Build history of the part. All positions in model axes, mm. A direction names the side the tool comes from. Coordinates: 2 decimals unless noted, no trailing zeros. Write each loop counter-clockwise with the first axis right and the second up, starting at its lowest first coordinate (ties: lowest second). Pieces come first, ordered by that corner, then holes.
Autodesk Inventor part; units mm, degrees
ref_plane "YZ Plane" through (0, 0, 0) normal (1, 0, 0) x (0, 1, 0)
ref_plane "XZ Plane" through (0, 0, 0) normal (0, 1, 0) x (-1, 0, 0)
ref_plane "XY Plane" through (0, 0, 0) normal (0, 0, 1) x (1, 0, 0)
sketch "Sketch1" plane through (0, 0, 0) normal (0, 0, 1) x (1, 0, 0)
  line L0 (0, 0) -> (63.5, 0)
  line L1 (63.5, 0) -> (63.5, 127)
  line L2 (63.5, 127) -> (0, 127)
  line L3 (0, 127) -> (0, 0)
  circle A0 centre (31.75, 95.25) radius 9.5
  circle A1 centre (31.75, 10.795) radius 2.6543
  circle A2 centre (31.75, -14.605) radius 2.6543
  line L4 (31.75, 115.6989) -> (31.75, 0)
  circle A3 centre (31.75, -40.005) radius 2.6543
  line L5 (44.45, 39.5543) -> (44.45, -52.705)
  line L6 (44.45, -52.705) -> (19.05, -52.705)
  line L7 (19.05, -52.705) -> (19.05, 39.5543)
  line L8 (44.45, 39.5543) -> (19.05, 39.5543)
  line L9 (0, 30.254) -> (63.5, 30.254)
  point P0 (44.45, 0)
  point P1 (19.05, 0)
  point P2 (31.75, -52.705)
  dimension "d0" = 63.5
  dimension "d1" = 127
  dimension "d2" = 19
  dimension "d3" = 5.3086
  dimension "d4" = 5.3086
  dimension "d5" = 31.75
  dimension "d6" = 116.205
  dimension "d14" = 25.4
  dimension "d15" = 25.4
  dimension "d17" = 25.4
  dimension "d20" = 39.5543
  dimension "d21" = 12.7
extrude "Extrusion1" add sketch "Sketch1" along normal blind 3.302 contours L3 L9 L7 L0 | L7 L9 L4 A1 L0 | L0 L5 L6 L7 | L3 L2 L1 L9 L5 L8 L7 | L4 A1 L9 L5 L0 | L7 L8 L4 L9 | L5 L9 L1 L0 | L4 L8 L5 L9
fillet "Fillet1" radius 31.75 1 edges at (63.5, 127, 1.651)
fillet "Fillet2" radius 31.75 1 edges at (0, 127, 1.651)
fillet "Fillet3" radius 3.175 1 edges at (63.5, 0, 1.651)
fillet "Fillet4" radius 3.175 1 edges at (0, 0, 1.651)
fillet "Fillet5" radius 6.35 2 edges at (19.05, 0, 1.651) (44.45, 0, 1.651)
properties part number "Wrist plate"
1. Saw through at C-C on x = 58.5. List the corners of the cut face in (y, z), plus the area to 3 significant figures.
Computed values:
outline: (0, 0) - (112.35, 0) - (112.35, 3.3) - (0, 3.3) - close
area: 371 mm2
2. Saw through at B-B on y = -30. List the corners of the cut face in (x, z).
Computed values:
outline: (19.05, 0) - (44.45, 0) - (44.45, 3.3) - (19.05, 3.3) - close
3. Flat gauge pins, fed straight in: pin 1 (1 mm diameter, centred on x = 10, z = 1.5, fed in from -Y); pin 2 (1.7 mm diameter, centred on y = -18, z = 2.5, fed in from -X); pin 3 (1.5 mm diameter, centred on x = 55, z = 2.5, fed in from +Y). Where does each tip first touch, or does it go through?
Computed values:
pin 1: stops at y = 0
pin 2: stops at x = 19.05
pin 3: stops at y = 117.65
4. Saw through at A-A on z = 2.65. State how many separate pieces and enclosed holes the cut face has, plus the area to 3 significant figures.
Computed values:
separate pieces: 1
enclosed holes: 4
area: 8,630 mm2
5. Probe line 1 along Y through (x, z) = (31.75, 1.7) (3 decimals); line 2 along Y through (x, z) = (32, 1.9) (1 decimal); line 3 along X through (y, z) = (96, 2.7). List the from-to ranges inside material, lowest first.
Computed values:
line 1: y = -52.705 to -42.659, -37.351 to -17.259, -11.951 to 8.141, 13.449 to 85.75, 104.75 to 127
line 2: y = -52.7 to -42.6, -37.4 to -17.2, -12 to 8.2, 13.4 to 85.8, 104.7 to 127
line 3: x = 0.01 to 22.28, 41.22 to 63.49
6. 3-axis set-ups, long thin cutter, end or side, ignore diameter. For faces 1 (the face through (9.5, 117.9, 1.7)), 2 (the face through (44.45, -29, 2)), 3 (the face through (19.05, -30, 2)): which of +Z, -Z, +X, -X, +Y, -Y reach the whole face in a straight line?
Computed values:
face 1: +Z, -Z, -X, +Y
face 2: +Z, -Z, +X, -Y
face 3: +Z, -Z, -X, -Y
